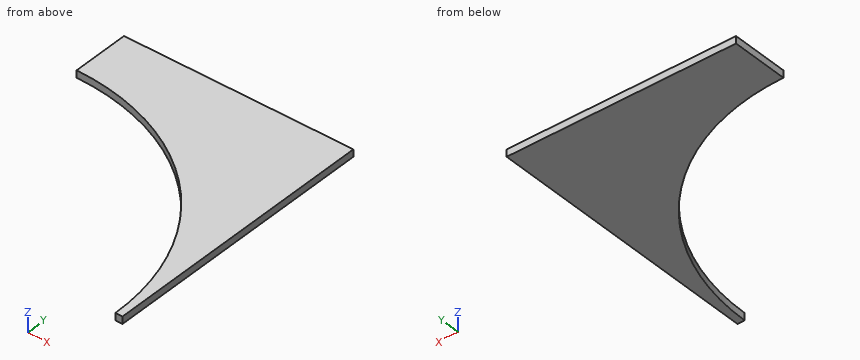
```python
from build123d import *

# Parameters (mm, degrees)
BOSS_EXTRUDE1_DEPTH = 3.175


with BuildPart() as part:
    # Sketch1 → Boss-Extrude1 (new body)
    with BuildSketch(Plane.XY):
        with BuildLine():
            Line((-71.953806461, 91.039951247), (29.646193539, 91.039951247))
            Line((29.646193539, 91.039951247), (29.646193539, -32.785048753))
            Line((29.646193539, -32.785048753), (26.471193539, -32.785048753))
            ThreePointArc((26.471193539, -32.785048753), (-2.356821523, 36.811936186), (-71.953806461, 65.639951247))
            Line((-71.953806461, 65.639951247), (-71.953806461, 91.039951247))
        make_face()
    extrude(amount=-BOSS_EXTRUDE1_DEPTH)


solid = part.part
```
Geometry check sheet. Reference: the model listing, model coordinates, mm. Coordinates: 2 decimals unless noted, no trailing zeros. Order: outer loops, then holes, each group sorted by start corner. A loop starts at its lowest first (then second) coordinate and runs counter-clockwise, first axis right, second up.
Q1. Thickness scan on probe 1 along Y at (x, z) = (-63, -1); probe 2 along X at (y, z) = (44, -2.6); probe 3 along X at (y, z) = (25, -1.05). Record the ranges inside material, lowest first.
Reply:
probe 1: y = 65.23 to 91.04
probe 2: x = -10.38 to 29.65
probe 3: x = 7.72 to 29.65
Q2. Sectioned sample at A-A on z = -1.5. Record the cut outline in (x, y) (3 decimals), and give its area (3 significant figures).
Reply:
outline: (-71.954, 65.64) arc R98.425 cw to (26.471, -32.785) - (29.646, -32.785) - (29.646, 91.04) - (-71.954, 91.04) - close
area: 4,970 mm2
Q3. Sectioned sample at B-B on y = 30.5. Record the cut outline in (x, z) (3 decimals), and give its area (3 significant figures).
Reply:
outline: (3.428, -3.175) - (29.646, -3.175) - (29.646, 0) - (3.428, 0) - close
area: 83.2 mm2
Q4. Sectioned sample at C-C on x = -43. Record the cut outline in (y, z) (3 decimals), and give its area (3 significant figures).
Reply:
outline: (61.285, -3.175) - (91.04, -3.175) - (91.04, 0) - (61.285, 0) - close
area: 94.5 mm2
